from build123d import *

# Parameters (mm, degrees)
CROQUIS1_W              = 15
CROQUIS1_H              = 15
CROQUIS1_W_2            = 4
CROQUIS1_W_3            = 16
CROQUIS1_R              = 1.5
SALIENTE_EXTRUIR1_DEPTH = 4
CROQUIS2_W              = 4
CROQUIS2_H              = 15
SALIENTE_EXTRUIR2_DEPTH = 60
CROQUIS3_W              = 15
CROQUIS3_H              = 15
SALIENTE_EXTRUIR3_DEPTH = 20
CROQUIS9_R              = 2.85
CORTAR_EXTRUIR3_DEPTH   = 1.65
CORTAR_EXTRUIR4_REACH   = 76.471
CROQUIS4_R              = 1.5
CROQUIS4_3_R            = 1.5
CORTAR_EXTRUIR5_DEPTH   = 2
CROQUIS10_W             = 15
CROQUIS10_H             = 15
CORTAR_EXTRUIR6_DEPTH   = 4
CROQUIS11_R             = 1.5
CORTAR_EXTRUIR7_DEPTH   = 6
CROQUIS12_R             = 2.75
CORTAR_EXTRUIR9_DEPTH   = 1


with BuildPart() as part:
    # Croquis1 → Saliente-Extruir1 (new body)
    # profile 1 of 3: a face of its own
    with BuildSketch(Plane.XY):
        with Locations((11.5, 7.5)):
            Rectangle(CROQUIS1_W, CROQUIS1_H)
    # profile 2 of 3: a face of its own
    with BuildSketch(Plane.XY):
        with Locations((2, 7.5)):
            Rectangle(CROQUIS1_W_2, CROQUIS1_H)
    # profile 3 of 3: a face of its own
    with BuildSketch(Plane.XY):
        with Locations((27, 7.5)):
            Rectangle(CROQUIS1_W_3, CROQUIS1_H)
        with Locations((23, 11.25)):
            Circle(CROQUIS1_R, mode=Mode.SUBTRACT)
        with Locations((31, 11.25)):
            Circle(CROQUIS1_R, mode=Mode.SUBTRACT)
        with Locations((31, 3.75)):
            Circle(CROQUIS1_R, mode=Mode.SUBTRACT)
        with Locations((23, 3.75)):
            Circle(CROQUIS1_R, mode=Mode.SUBTRACT)
    extrude(amount=SALIENTE_EXTRUIR1_DEPTH)

    # Croquis2 → Saliente-Extruir2 (add)
    with BuildSketch(Plane.XY.offset(4)):
        with Locations((2, 7.5)):
            Rectangle(CROQUIS2_W, CROQUIS2_H)
    extrude(amount=SALIENTE_EXTRUIR2_DEPTH)

    # Croquis3 → Saliente-Extruir3 (add)
    with BuildSketch(Plane.XY.offset(4)):
        with Locations((11.5, 7.5)):
            Rectangle(CROQUIS3_W, CROQUIS3_H)
    extrude(amount=SALIENTE_EXTRUIR3_DEPTH)

    # Croquis9 → Cortar-Extruir3 (cut)
    with BuildSketch(Plane.XY.offset(4)):
        with Locations((23, 3.75)):
            Circle(CROQUIS9_R)
        with Locations((31, 3.75)):
            Circle(CROQUIS9_R)
        with Locations((23, 11.25)):
            Circle(CROQUIS9_R)
        with Locations((31, 11.25)):
            Circle(CROQUIS9_R)
    extrude(amount=-CORTAR_EXTRUIR3_DEPTH, mode=Mode.SUBTRACT)

    # Croquis4 → Cortar-Extruir4 (cut, up to next)
    with BuildSketch(Plane(origin=(0, 0, 0), x_dir=(0, 0, -1), z_dir=(1, 0, 0)), mode=Mode.PRIVATE) as cortar_extruir4_sk1:
        with Locations(Location((-59.52, 10.8, 0), (0, 0, 180))):
            Circle(CROQUIS4_R)
    cortar_extruir4_tool1 = extrude(cortar_extruir4_sk1.sketch, amount=CORTAR_EXTRUIR4_REACH, mode=Mode.PRIVATE) & part.part
    # Croquis4 → Cortar-Extruir4 (cut, up to next)
    with BuildSketch(Plane(origin=(0, 0, 0), x_dir=(0, 0, -1), z_dir=(1, 0, 0)), mode=Mode.PRIVATE) as cortar_extruir4_sk2:
        with Locations(Location((-52.48, 4.2, 0), (0, 0, 180))):
            Circle(CROQUIS4_R)
    cortar_extruir4_tool2 = extrude(cortar_extruir4_sk2.sketch, amount=CORTAR_EXTRUIR4_REACH, mode=Mode.PRIVATE) & part.part
    add(cortar_extruir4_tool1.solids().sort_by_distance((0, 10.8, 59.52))[0], mode=Mode.SUBTRACT)
    add(cortar_extruir4_tool2.solids().sort_by_distance((0, 4.2, 52.48))[0], mode=Mode.SUBTRACT)

    # Croquis4<3> → Cortar-Extruir5 (cut)
    # profile 1 of 2: a face of its own
    with BuildSketch(Plane(origin=(0, 0, 0), x_dir=(0, 0, -1), z_dir=(1, 0, 0))):
        Polygon((-59.52, 13.975426481), (-62.27, 12.38771324), (-62.27, 9.21228676), (-59.52, 7.624573519), (-56.77, 9.21228676), (-56.77, 12.38771324), align=None)
        with Locations(Location((-59.52, 10.8, 0), (0, 0, 180))):
            Circle(CROQUIS4_3_R, mode=Mode.SUBTRACT)
    # profile 2 of 2: a face of its own
    with BuildSketch(Plane(origin=(0, 0, 0), x_dir=(0, 0, -1), z_dir=(1, 0, 0))):
        Polygon((-52.48, 7.375426481), (-55.23, 5.78771324), (-55.23, 2.61228676), (-52.48, 1.024573519), (-49.73, 2.61228676), (-49.73, 5.78771324), align=None)
        with Locations(Location((-52.48, 4.2, 0), (0, 0, 180))):
            Circle(CROQUIS4_3_R, mode=Mode.SUBTRACT)
    extrude(amount=CORTAR_EXTRUIR5_DEPTH, mode=Mode.SUBTRACT)

    # Croquis10 → Cortar-Extruir6 (cut)
    with BuildSketch(Plane(origin=(0, 0, 0), x_dir=(1, 0, 0), z_dir=(0, 1, 0))):
        with Locations((11.5, -16.5)):
            Rectangle(CROQUIS10_W, CROQUIS10_H)
    extrude(amount=CORTAR_EXTRUIR6_DEPTH, mode=Mode.SUBTRACT)

    # Croquis11 → Cortar-Extruir7 (cut)
    with BuildSketch(Plane(origin=(0, 4, 0), x_dir=(-1, 0, 0), z_dir=(0, -1, 0))):
        with Locations(Location((-8.2, -13.2, 0), (0, 0, 90))):
            Circle(CROQUIS11_R)
        with Locations(Location((-14.8, -19.8, 0), (0, 0, 90))):
            Circle(CROQUIS11_R)
    extrude(amount=-CORTAR_EXTRUIR7_DEPTH, mode=Mode.SUBTRACT)

    # Croquis12 → Cortar-Extruir9 (cut)
    with BuildSketch(Plane.XZ.offset(-4)):
        with Locations(Location((8.2, 13.2, 0), (0, 0, 270))):
            Circle(CROQUIS12_R)
        with Locations(Location((14.8, 19.8, 0), (0, 0, 270))):
            Circle(CROQUIS12_R)
    extrude(amount=-CORTAR_EXTRUIR9_DEPTH, mode=Mode.SUBTRACT)


solid = part.part
CAD build for the part. Positions are in the model's coordinates, mm. A direction names the side the tool comes from. Coordinates: 2 decimals unless noted, no trailing zeros. Write each loop counter-clockwise with the first axis right and the second up, starting at its lowest first coordinate (ties: lowest second). Pieces come first, ordered by that corner, then holes. Notation, with made-up numbers: (-25.75, 74.25) - (7.25, 74.25) arc R32 ccw to (7.25, 108.25) - close; hole circle Ø8 at (23, 49.5). An arc over 180 degrees is marked (long way). Use a Markdown table: item, result. Add a question column.
Item 1: Band-saw the part on C-C, the plane x = 15.5. Give the cut face in (y, z).
Item 2: Band-saw the part on D-D, the plane z = 48. Give the cut face in (x, y), and give its area (3 significant figures).
Item 3: Drill centre lines: L1, parallel to Y at x = 31, z = 1.3; L2, parallel to X at y = 11.25, z = 1.4; L3, parallel to X at y = 4.25, z = 13. Where is each one in solid material? Low to high. Write a range as from..to.
Item 4: Band-saw the part on B-B, the plane z = 13.2. Give the cut face in (x, y).
Item 5: Flat gauge pins, fed straight in: pin 1 (4.5 mm diameter, centred on x = 23, y = 3.75, fed in from +Z); pin 2 (6 mm diameter, centred on x = 13, y = 9.5, fed in from -Z); pin 3 (2 mm diameter, centred on y = 2, z = 23.5, fed in from +X); pin 4 (1.6 mm diameter, centred on y = 4, z = 53.5, fed in from -X). Where does each tip first touch, or does it go through?
Item 6: Band-saw the part on A-A, the plane x = 23. Give the cut face in (y, z), and give its area (3 significant figures).
Item 7: 3-axis set-ups, long thin cutter, end or side, ignore diameter. For faces 1 (the face through (13.336, 7.465, 20.125)), 2 (the face through (17, 8, 0)), 3 (the face through (22.629, 14.076, 3.187)), 4 (the face through (11, 10, 24)), 5 (the face through (0.99, 6.59, 53.84)): which of +Z, -Z, +X, -X, +Y, -Y reach the whole face in a straight line?
Item 8: Mould opens along Y. For faces 6 (the face through (1, 11, 56.77)), 7 (the face through (2, 8, 64)), 8 (the face through (13.6, 5, 18.6)), 9 (the face through (29.5, 11.3, 1.2)) say: pulls with the +Y half, pulls with the -Y half, needs draft (parallel to the pull), parting line crosses it, or undercut.
Numbers:
| question | item | result |
|---|---|---|
| 1 | outline | (0, 0) - (15, 0) - (15, 24) - (4, 24) - (4, 22.46) - (5, 22.46) - (5, 21.13) - (10, 21.13) - (10, 18.47) - (5, 18.47) - (5, 17.14) - (4, 17.14) - (4, 9) - (0, 9) - close |
| 2 | outline | (0, 0) - (4, 0) - (4, 15) - (0, 15) - close |
| 2 | area | 60.0 mm2 |
| 3 | L1 | 0..2.25, 5.25..9.75, 12.75..15 |
| 3 | L2 | 0..21.5, 24.5..29.5, 32.5..35 |
| 3 | L3 | 0..5.46, 10.94..19 |
| 4 | outline | (0, 0) - (4, 0) - (4, 4) - (5.45, 4) - (5.45, 5) - (6.7, 5) - (6.7, 10) - (9.7, 10) - (9.7, 5) - (10.95, 5) - (10.95, 4) - (19, 4) - (19, 15) - (0, 15) - close |
| 5 | pin 1 | z = 2.35 |
| 5 | pin 2 | z = 0 |
| 5 | pin 3 | x = 4 |
| 5 | pin 4 | x = 2 |
| 6 | outline | (0, 0) - (2.25, 0) - (2.25, 2.35) - (0.9, 2.35) - (0.9, 4) - (0, 4) - close; (5.25, 0) - (9.75, 0) - (9.75, 2.35) - (8.4, 2.35) - (8.4, 4) - (6.6, 4) - (6.6, 2.35) - (5.25, 2.35) - close; (12.75, 0) - (15, 0) - (15, 4) - (14.1, 4) - (14.1, 2.35) - (12.75, 2.35) - close |
| 6 | area | 27.1 mm2 |
| 7 | face 1 | -Y |
| 7 | face 2 | -Z, +X, -X, +Y, -Y |
| 7 | face 3 | +Z |
| 7 | face 4 | +Z, +X, +Y, -Y |
| 7 | face 5 | -X |
| 8 | face 6 | undercut |
| 8 | face 7 | needs draft |
| 8 | face 8 | pulls with the -Y half |
| 8 | face 9 | undercut |
